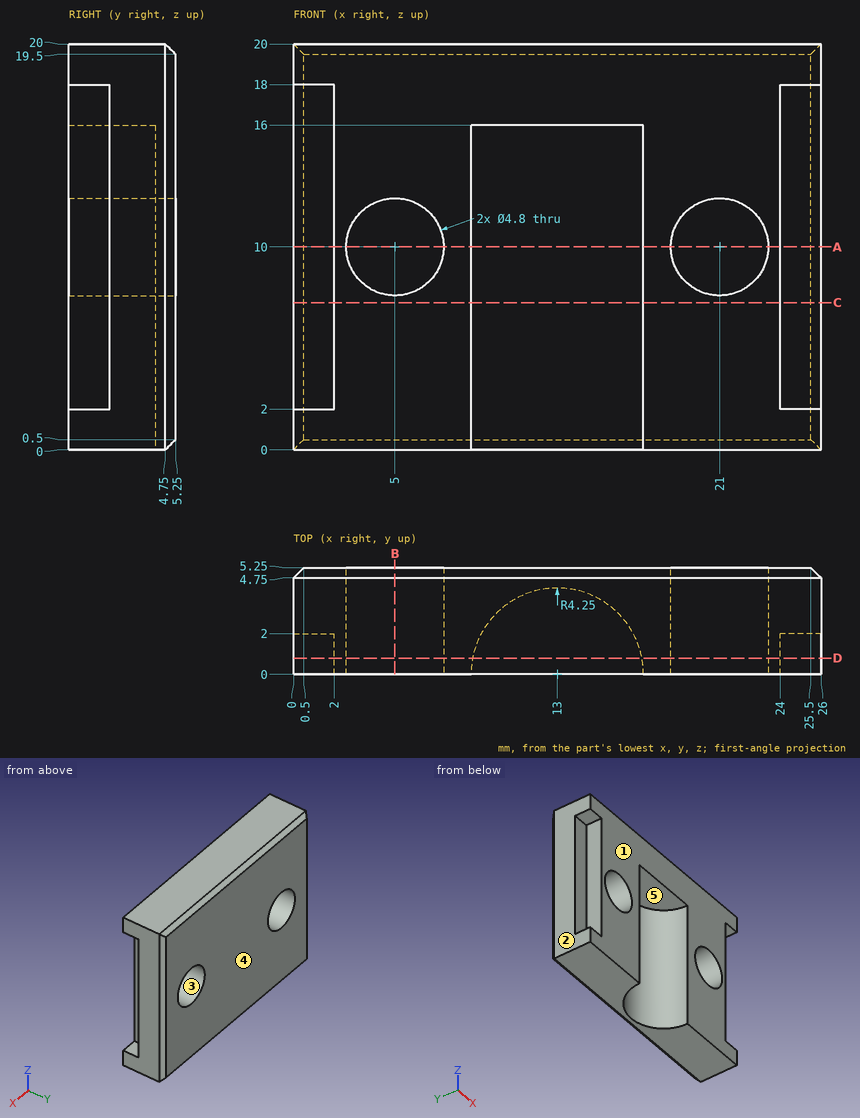
For this review, use the dimensioned drawing (mm, ordinates from the lowest corner) and the shaded views. A direction names the side the tool comes from. Coordinates: 2 decimals unless noted, no trailing zeros. Write each loop counter-clockwise with the first axis right and the second up, starting at its lowest first coordinate (ties: lowest second). Pieces come first, ordered by that corner, then holes. Notation, with made-up numbers: (-33, -39) - (19, -39) arc R21 ccw to (19, -25) - close; hole circle Ø9 at (59, 71). An arc over 180 degrees is marked (long way). One line per item, written item: value.
1) To check wall thickness, follow probe 1 along Z at (x, y) = (5, 1.4); probe 2 along X at (y, z) = (2.2, 9.5); probe 3 along X at (y, z) = (1.4, 10). State the ranges of each line that lie inside material, in increasing order.
Answer sheet:
probe 1: z = 0 to 7.6, 12.4 to 20
probe 2: x = 0 to 2.65, 7.35 to 9.36, 16.64 to 18.65, 23.35 to 26
probe 3: x = 2 to 2.6, 7.4 to 8.99, 17.01 to 18.6, 23.4 to 24
2) Add section C-C (z = 7.25). State the section outline as (x, y) points, plus the area to 3 significant figures.
Answer sheet:
outline: (0, 2) - (2, 2) - (2, 0) - (8.75, 0) arc R4.25 cw to (17.25, 0) - (24, 0) - (24, 2) - (26, 2) - (26, 4.75) - (25.5, 5.25) - (0.5, 5.25) - (0, 4.75) - close
area: 99.9 mm2
3) Insertion check: pin 1 (2 mm diameter, centred on y = 0.5, z = 12.5, fed in from -X); pin 2 (0.6 mm diameter, centred on x = 25, z = 14, fed in from -Y); pin 3 (2 mm diameter, centred on x = 14, y = 2.5, fed in from -Z). Each pin has a flat end and moves straight along its axis. Give the tip position at first contact, or say it passes through.
Answer sheet:
pin 1: stops at x = 2
pin 2: stops at y = 2
pin 3: stops at z = 16
4) Add section B-B (x = 5). State the section outline as (y, z) points.
Answer sheet:
outline: (0, 0) - (4.75, 0) - (5.25, 0.5) - (5.25, 7.6) - (0, 7.6) - close; (0, 12.4) - (5.25, 12.4) - (5.25, 19.5) - (4.75, 20) - (0, 20) - close
5) Add section D-D (y = 0.8). State the section outline as (x, z) points.
Answer sheet:
outline: (0, 0) - (8.83, 0) - (8.83, 16) - (17.17, 16) - (17.17, 0) - (26, 0) - (26, 2) - (24, 2) - (24, 18) - (26, 18) - (26, 20) - (0, 20) - (0, 18) - (2, 18) - (2, 2) - (0, 2) - close; hole circle Ø4.8 at (5, 10); hole circle Ø4.8 at (21, 10)
6) Mouldability with a two-part tool opening along X and no side actions: class the marked faces 1, 2 and 3 as +X half, -X half, draft (parallel to the pull), parting line (faces both ways), or undercut.
Answer sheet:
face 1: draft
face 2: -X half
face 3: undercut
7) Add section A-A (z = 10). State the section outline as (x, y) points, plus the area to 3 significant figures.
Answer sheet:
outline: (0, 2) - (2, 2) - (2, 0) - (2.6, 0) - (2.6, 5.25) - (0.5, 5.25) - (0, 4.75) - close; (7.4, 0) - (8.75, 0) arc R4.25 cw to (17.25, 0) - (18.6, 0) - (18.6, 5.25) - (7.4, 5.25) - close; (23.4, 0) - (24, 0) - (24, 2) - (26, 2) - (26, 4.75) - (25.5, 5.25) - (23.4, 5.25) - close
area: 49.5 mm2
8) For the marked faces 4 and 5, list the 3-axis set-ups (+Z, -Z, +X, -X, +Y, -Y) from which the entire face can be reached by the end or side of a thin tool; tool diameter is ignored.
Answer sheet:
face 4: +Z, -Z, +X, -X, +Y
face 5: -Z, -Y
